```python
from build123d import *

# Parameters (mm, degrees)
BASENUTSKE_R  = 1.25
BASENUT_DEPTH = 2.3


with BuildPart() as part:
    # BaseNutSke → BaseNut (new body)
    with BuildSketch(Plane.XY):
        Polygon((2.705, 1.561732478), (2.705, -1.561732478), (0, -3.123464956), (-2.705, -1.561732478), (-2.705, 1.561732478), (0, 3.123464956), align=None)
        Circle(BASENUTSKE_R, mode=Mode.SUBTRACT)
    extrude(amount=-BASENUT_DEPTH)

    # Sketch3 → Double-Chamfer (revolve, cut)
    with BuildSketch(Plane(origin=(0, 0, 0), x_dir=(0, 0, -1), z_dir=(1, 0, 0))):
        Polygon((2.3, 2.705), (2.058399145, 3.123464956), (2.058399145, 13.123464956), (12.3, 13.123464956), (12.3, 2.705), align=None)
        Polygon((0.241600855, 13.123464956), (-10, 13.123464956), (-10, 2.705), (0, 2.705), (0.241600855, 3.123464956), align=None)
    revolve(axis=Axis((0, 0, 0), (0, 0, -1)), mode=Mode.SUBTRACT)

    # Sketch5 (on Right Plane) → EndChamfer (revolve, cut)
    with BuildSketch(Plane(origin=(0, 0, 0), x_dir=(0, 0, -1), z_dir=(1, 0, 0)), mode=Mode.PRIVATE) as endchamfer_sk:
        Polygon((2.2746, 1.5), (2.082042927, 1.225), (2.3254, 1.225), (2.3254, 1.5), align=None)
        Polygon((-0.0508, 1.5), (0, 1.5), (0.192557073, 1.225), (-0.0508, 1.225), align=None)
    revolve(endchamfer_sk.sketch.rotate(Axis((0, 0, -25.037505729), (0, 0, -1)), 90), axis=Axis((0, 0, -25.037505729), (0, 0, -1)), mode=Mode.SUBTRACT)


solid = part.part
```
Work out the finished part from the listing and answer in its coordinate system (mm). Give positions to 0.01 mm unless a question says otherwise; leave off trailing zeros. Order: outer loops, then holes, each group sorted by start corner. A loop starts at its lowest first (then second) coordinate and runs counter-clockwise, first axis right, second up.
1. This flat-tipped pin is pushed along its axis until it touches: P1, Ø3, axis at x = 0, y = -2, coming from the +Z side. Where does it stop, or does it pass through?
Result sheet:
P1: stops at z = 0
2. Section A-A, the plane z = -1.55 is taken. Determine the outline of the cut face in (x, y) (3 decimals), and give its area (3 significant figures).
Result sheet:
outline: (-2.705, -1.562) - (0, -3.123) - (2.705, -1.562) - (2.705, 1.562) - (0, 3.123) - (-2.705, 1.562) - close; hole circle Ø2.5 at (0, 0)
area: 20.4 mm2
3. Straight lines are drawn through the part: L1, parallel to X at y = -0.75, z = -1.6 (3 decimals); L2, parallel to Y at x = 1.05, z = -0.75; L3, parallel to X at y = 2.75, z = -1.85. For each, find the intervals that lie inside material, in ascending order.
Result sheet:
L1: x = -2.705 to -1, 1 to 2.705
L2: y = -2.52 to -0.68, 0.68 to 2.52
L3: x = -0.65 to 0.65
4. The mould has two halves that part along Y. Classify faces 1 (the flat face through (-1.334, -2.354, -1.134)), 2 (the flat face through (-1.2, -1.2, 0)), 3 (the cylindrical face through (-0.27, -1.22, -1.12)): released by +Y, released by -Y, zero draft, split by the parting line, or undercut.
Result sheet:
face 1: released by -Y
face 2: zero draft
face 3: undercut
